```python
from build123d import *

# Parameters (mm, degrees)
SKETCH_1_R          = 60
EXTRUDE_1_DEPTH     = 4
SKETCH_2_R          = 12.5875
SKETCH_2_R_2        = 1
SKETCH_2_R_3        = 2
CUT_EXTRUDE_2_DEPTH = 4
EXTRUDE_START       = -2.85
SKETCH_2_4_R        = 4.5
EXTRUDE_2_DEPTH     = 2.85


with BuildPart() as part:
    # 草圖1 → 填料-伸長1 (new body)
    with BuildSketch(Plane.XY):
        Circle(SKETCH_1_R)
    extrude(amount=EXTRUDE_1_DEPTH)

    # 草圖2 → 除料-伸長2 (cut)
    with BuildSketch(Plane.XY):
        with BuildLine():
            ThreePointArc((-1.46, 1.942498391), (-2.43, 0), (-1.46, -1.942498391))
            Line((-1.46, -1.942498391), (1.46, -1.942498391))
            ThreePointArc((1.46, -1.942498391), (2.43, 0), (1.46, 1.942498391))
            Line((1.46, 1.942498391), (-1.46, 1.942498391))
        make_face()
        with Locations((-40.5, 0)):
            Circle(SKETCH_2_R)
        with Locations((-20.25, 35.074028853)):
            Circle(SKETCH_2_R)
        with Locations((20.25, 35.074028853)):
            Circle(SKETCH_2_R)
        with Locations((40.5, 0)):
            Circle(SKETCH_2_R)
        with Locations((20.25, -35.074028853)):
            Circle(SKETCH_2_R)
        with Locations((-20.25, -35.074028853)):
            Circle(SKETCH_2_R_2)
        with Locations((-17.1, -29.618068809)):
            Circle(SKETCH_2_R_3)
        with Locations((-22.555960044, -26.468068809)):
            Circle(SKETCH_2_R_2)
        with Locations((-11.644039956, -32.768068809)):
            Circle(SKETCH_2_R_2)
        with Locations((-17.944039956, -43.679988897)):
            Circle(SKETCH_2_R_2)
        with Locations((-28.855960044, -37.379988897)):
            Circle(SKETCH_2_R_2)
        with Locations((-14.794039956, -38.224028853)):
            Circle(SKETCH_2_R_3)
        with Locations((-25.705960044, -31.924028853)):
            Circle(SKETCH_2_R_3)
        with Locations((-23.4, -40.529988897)):
            Circle(SKETCH_2_R_3)
        with Locations((-31.161920088, -28.774028853)):
            Circle(SKETCH_2_R_2)
        with Locations((-13.95, -24.162108766)):
            Circle(SKETCH_2_R_2)
        with Locations((-9.338079912, -41.374028853)):
            Circle(SKETCH_2_R_2)
        with Locations((-26.55, -45.985948941)):
            Circle(SKETCH_2_R_2)
    extrude(amount=CUT_EXTRUDE_2_DEPTH, mode=Mode.SUBTRACT)

    # 草圖2<4> → 填料-伸長2 (add)
    with BuildSketch(Plane.XY.offset(EXTRUDE_START)):
        Circle(SKETCH_2_4_R)
        with BuildLine():
            ThreePointArc((1.46, -1.942498391), (2.43, 0), (1.46, 1.942498391))
            Line((1.46, 1.942498391), (-1.46, 1.942498391))
            ThreePointArc((-1.46, 1.942498391), (-2.43, 0), (-1.46, -1.942498391))
            Line((-1.46, -1.942498391), (1.46, -1.942498391))
        make_face(mode=Mode.SUBTRACT)
    extrude(amount=EXTRUDE_2_DEPTH)


solid = part.part
```
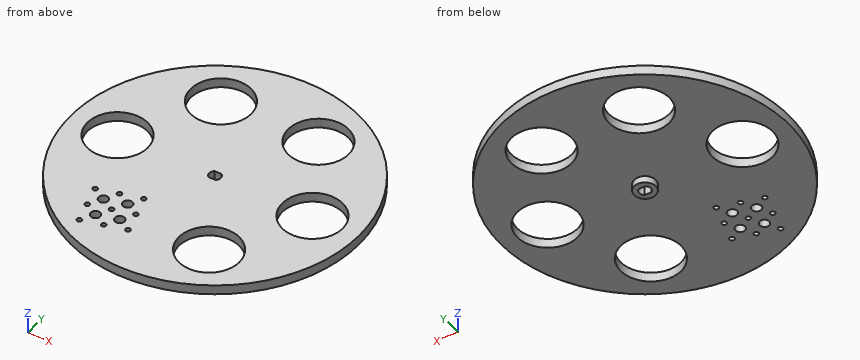
Design review of the part built by this model. Coordinates are the model's own, in mm. Give positions to 0.01 mm unless a question says otherwise; leave off trailing zeros. Order: outer loops, then holes, each group sorted by start corner. A loop starts at its lowest first (then second) coordinate and runs counter-clockwise, first axis right, second up. Notation, with made-up numbers: (45.5, -2) -> (90.5, -2) arc R28 cw to (90.5, 18) -> close; hole circle Ø9 at (6.5, 70). An arc over 180 degrees is marked (long way). Write item = value, one per line. Start each with the question number.
(1) We need section A-A on x = 20.25. Write out the cut boundary in (y, z).
(2) We need section D-D on y = 51. Write out the cut boundary in (x, z).
(3) For pin 1 (1.5 mm diameter, centred on x = 0, z = 1, fed in from -Y); pin 2 (3.5 mm diameter, centred on x = -23.4, y = -40.53, fed in from -Z); pin 3 (3 mm diameter, centred on x = 0.5, z = 0.5, fed in from +Y); pin 4 (2 mm diameter, centred on y = 26.5, z = 2, fed in from -X), all flat-tipped, find the tip position at first contact; note any pin that passes through.
(4) We need section B-B on x = 36. Write out the cut boundary in (y, z).
(5) To check wall thickness, follow line 1 along X through (y, z) = (44, 1.5); line 2 along X through (y, z) = (-29.5, 3.25); line 3 along Y through (x, z) = (-20.25, 2.1). State the ranges of each line that lie inside material, in increasing order.
(6) We need section C-C on z = 2. State how many separate pieces and enclosed holes the cut face has, plus the area to 3 significant figures.
Numbers:
q1.outline = (-56.48, 0) -> (-47.66, 0) -> (-47.66, 4) -> (-56.48, 4) -> close; (-22.49, 0) -> (22.49, 0) -> (22.49, 4) -> (-22.49, 4) -> close; (47.66, 0) -> (56.48, 0) -> (56.48, 4) -> (47.66, 4) -> close
q2.outline = (-31.61, 0) -> (31.61, 0) -> (31.61, 4) -> (-31.61, 4) -> close
q3.pin_1 = -60
q3.pin_2 = through
q3.pin_3 = 60
q3.pin_4 = -54.31
q4.outline = (-48, 0) -> (-11.76, 0) -> (-11.76, 4) -> (-48, 4) -> close; (11.76, 0) -> (48, 0) -> (48, 4) -> (11.76, 4) -> close
q5.line_1 = -40.79 to -29.13, -11.37 to 11.37, 29.13 to 40.79
q5.line_2 = -52.25 to -31.85, -30.47 to -19.1, -15.1 to 8.96, 31.54 to 52.25
q5.line_3 = -56.48 to -36.07, -34.07 to 22.49, 47.66 to 56.48
q6.separate_pieces = 1
q6.enclosed_holes = 19
q6.area = 8,730 mm^2
